Geometry: final body of the model. Coordinates: model frame, mm. A direction names the side the tool comes from. Round coordinates to 2 decimals unless told otherwise and drop trailing zeros. Write each loop counter-clockwise with the first axis right and the second up, starting at its lowest first coordinate (ties: lowest second). Pieces come first, ordered by that corner, then holes. Notation, with made-up numbers: (28.5, 35.25) - (59.5, 35.25) arc R5 ccw to (59.5, 41.25) - close; hole circle Ø9 at (73.5, -18). An arc over 180 degrees is marked (long way). Use a Markdown table: item, result. Add a question column.
```python
from build123d import *

# Parameters (mm, degrees)
BOSS_EXTRU_1_DEPTH      = 3
ESQUISSE21_W            = 11.4
ESQUISSE21_H            = 11.4
ENL_V_MAT_EXTRU_3_DEPTH = 4
D_GAGEMENT_M41_D        = 4.5
D_GAGEMENT_M42_D        = 4.5
D_GAGEMENT_M201_D       = 22
ENL_V_MAT_EXTRU_4_DEPTH = 4


with BuildPart() as part:
    # Esquisse1 → Boss.-Extru.1 (new body)
    with BuildSketch(Plane.XY):
        with BuildLine():
            Line((-145, 85), (-109.886246, 120.113754))
            Line((-109.886246, 120.113754), (109.886246, 120.113754))
            Line((109.886246, 120.113754), (145, 85))
            Line((145, 85), (145, -85))
            Line((145, -85), (109.886246, -120.113754))
            Line((109.886246, -120.113754), (104.886246, -120.113754))
            ThreePointArc((104.886246, -120.113754), (0, -20), (-104.886246, -120.113754))
            Line((-104.886246, -120.113754), (-109.886246, -120.113754))
            Line((-109.886246, -120.113754), (-145, -85))
            Line((-145, -85), (-145, 85))
        make_face()
    extrude(amount=BOSS_EXTRU_1_DEPTH)

    # Esquisse21 → Enlèv. mat.-Extru.3 (cut, through all)
    with BuildSketch(Plane.XY.offset(3)):
        with Locations((-139.3, 79.3)):
            Rectangle(ESQUISSE21_W, ESQUISSE21_H)
        with Locations((139.3, 79.3)):
            Rectangle(ESQUISSE21_W, ESQUISSE21_H)
        with Locations((-139.3, -79.3)):
            Rectangle(ESQUISSE21_W, ESQUISSE21_H)
        with Locations((139.3, -79.3)):
            Rectangle(ESQUISSE21_W, ESQUISSE21_H)
    extrude(amount=-ENL_V_MAT_EXTRU_3_DEPTH, mode=Mode.SUBTRACT)

    # Dégagement M41 (through all)
    with Locations(Plane(origin=(0, 0, 0), x_dir=(-1, 0, 0), z_dir=(0, 0, -1))):
        with Locations((-139.3, 55), (-139.3, 0), (-139.3, -55), (139.3, 55), (139.3, 0), (139.3, -55)):
            Hole(D_GAGEMENT_M41_D / 2)

    # Dégagement M42 (through all)
    with Locations(Plane.XY.offset(3)):
        with Locations((-60, 90.713754), (0, 90.713754), (60, 90.713754)):
            Hole(D_GAGEMENT_M42_D / 2)

    # Dégagement M201 (through all)
    with Locations(Plane(origin=(0, 0, 0), x_dir=(-1, 0, 0), z_dir=(0, 0, -1))):
        with Locations((-115, 85.113754), (-115, -85.113754), (115, 85.113754), (115, -85.113754)):
            Hole(D_GAGEMENT_M201_D / 2)

    # Esquisse46 → Enlèv. mat.-Extru.4 (cut, through all)
    with BuildSketch(Plane(origin=(0, 0, 0), x_dir=(-1, 0, 0), z_dir=(0, 0, -1))):
        with BuildLine():
            Line((-25, 50.113754), (25, 50.113754))
            ThreePointArc((25, 50.113754), (45, 30.113754), (25, 10.113754))
            Line((25, 10.113754), (-25, 10.113754))
            ThreePointArc((-25, 10.113754), (-45, 30.113754), (-25, 50.113754))
        make_face()
    extrude(amount=-ENL_V_MAT_EXTRU_4_DEPTH, mode=Mode.SUBTRACT)


solid = part.part
```
1) Section D-D, the plane x = 72. Return the cut outline in (y, z), then the cut area to 3 significant figures.
2) Draft query along Y for faces 3 (the cylindrical face through (-126, -85, 2)), 4 (the flat face through (2, 2, 3)), 5 (the flat face through (-127, -103, 1)). Return one class per face: released by +Y, released by -Y, zero draft, split by the parting line, or undercut.
3) Material intervals for L1, parallel to Y at x = 139.3, z = 1.5; L2, parallel to X at y = -92, z = 1.2; L3, parallel to X at y = -87, z = 2.8, sorted ascending. Write a range as from..to.
4) Set-up query: faces 1 (the flat face through (2, 2, 0)), 2 (the cylindrical face through (-44.995, 30.554, 1.479)). Return all of +Z, -Z, +X, -X, +Y, -Y with unobstructed straight access to the full face (end or side cutting, diameter ignored); none if empty.
5) Section C-C, the plane z = 1.25. State how many separate pieces and enclosed holes the cut face has, then the cut area to 3 significant figures.
6) Section B-B, the plane y = 28.5. Return the cut outline in (x, z), then the cut area to 3 significant figures.
7) Pin query (flat end, axial travel): P1, Ø1.5, axis at x = 139, z = 1.5, coming from the +Y side; P2, Ø0.9, axis at y = 81, z = 1.5, coming from the -X side; P3, Ø0.9, axis at x = 137.5, z = 1, coming from the -Y side. Return the tip coordinate at first contact, or that it passes through.
8) Section A-A, the plane x = -115. Return the cut outline in (y, z), then the cut area to 3 significant figures.
Output values:
| question | item | result |
|---|---|---|
| 1 | outline | (-48.57, 0) - (120.11, 0) - (120.11, 3) - (-48.57, 3) - close |
| 1 | area | 506 mm^2 |
| 2 | face 3 | undercut |
| 2 | face 4 | zero draft |
| 2 | face 5 | released by -Y |
| 3 | L1 | y = -90.7..-85, -73.6..-57.25, -52.75..-2.25, 2.25..52.75, 57.25..73.6, 85..90.7 |
| 3 | L2 | x = -138..-123.58, -106.42..-99.68, 99.68..106.42, 123.58..138 |
| 3 | L3 | x = -143..-125.84, -104.16..-97.88, 97.88..104.16, 125.84..143 |
| 4 | face 1 | -Z, +X, -X, +Y, -Y |
| 4 | face 2 | +Z, -Z |
| 5 | separate pieces | 1 |
| 5 | enclosed holes | 14 |
| 5 | area | 45,500 mm^2 |
| 6 | outline | (-145, 0) - (-44.93, 0) - (-44.93, 3) - (-145, 3) - close; (44.93, 0) - (145, 0) - (145, 3) - (44.93, 3) - close |
| 6 | area | 600 mm^2 |
| 7 | P1 | stops at y = 91.75 |
| 7 | P2 | stops at x = -133.6 |
| 7 | P3 | stops at y = -92.95 |
| 8 | outline | (-115, 0) - (-96.11, 0) - (-96.11, 3) - (-115, 3) - close; (-74.11, 0) - (74.11, 0) - (74.11, 3) - (-74.11, 3) - close; (96.11, 0) - (115, 0) - (115, 3) - (96.11, 3) - close |
| 8 | area | 558 mm^2 |
